```python
from build123d import *

# Parameters (mm, degrees)
SKETCH1_W      = 60
SKETCH1_H      = 60
EXTRUDE1_DEPTH = 50
SKETCH2_W      = 30
SKETCH2_H      = 15
EXTRUDE2_DEPTH = 40
CHAMFER1_SIZE  = 10


with BuildPart() as part:
    # Sketch1 → Extrude1 (new body)
    with BuildSketch(Plane(origin=(0, 0, 0), x_dir=(1, 0, 0), z_dir=(0, 1, 0))):
        Rectangle(SKETCH1_W, SKETCH1_H)
    extrude(amount=EXTRUDE1_DEPTH)

    # Sketch2 → Extrude2 (cut)
    with BuildSketch(Plane(origin=(0, 50, 0), x_dir=(1, 0, 0), z_dir=(0, 1, 0))):
        with Locations((15, -22.5)):
            Rectangle(SKETCH2_W, SKETCH2_H)
    extrude(amount=-EXTRUDE2_DEPTH, mode=Mode.SUBTRACT)

    # Chamfer1
    chamfer1_edges = [part.edges().sort_by_distance(p)[0] for p in [
        (30, 50, -7.5),
    ]]
    chamfer(chamfer1_edges, length=CHAMFER1_SIZE)


solid = part.part
```
Build history of the part. All positions in model axes, mm. A direction names the side the tool comes from. Give positions to 0.01 mm unless a question says otherwise; leave off trailing zeros. Order: outer loops, then holes, each group sorted by start corner. A loop starts at its lowest first (then second) coordinate and runs counter-clockwise, first axis right, second up. Notation, with made-up numbers: M -33.5,-6.75 L 6.5,-6.75 A16 cw 6.5,-1.75 Z; hole C 86.5,0 d11. An arc over 180 degrees is marked long. Write item = value, one per line. Start each with the question number.
(1) Slice it at B-B on x = 9.5. Write the cut outline in (y, z), plus the area to 3 significant figures.
(2) Probe L1, parallel to Z at x = 1, y = 46; L2, parallel to X at y = 21, z = 23; L3, parallel to X at y = 45, z = 7. List the from-to ranges inside material, lowest first. Write a range as [from, to].
(3) Which spindle directions (+Z, -Z, +X, -X, +Y, -Y) get a long thin tool onto all of the face, cutting with end or side? Do faces 1 (the flat face through (30, 20, -6)), 2 (the flat face through (15, 30, 15)). Say none if no direction does.
(4) Slice it at C-C on x = 21. Write the cut outline in (y, z).
(5) Pin check, flat tips, straight feed: pin 1 Ø7.5 at (x, z) = (9, 25.5) entering from +Y; pin 2 Ø7.5 at (y, z) = (25.5, 19) entering from +X; pin 3 Ø12 at (x, y) = (21, 41.5) entering from +Z. Stop position of each tip, or through.
(6) Slice it at A-A on z = -2. Write the cut outline in (x, y).
Responses:
q1.outline = M 0,-30 L 50,-30 L 50,15 L 10,15 L 10,30 L 0,30 Z
q1.area = 2,400 mm2
q2.L1 = [-30, 15]
q2.L2 = [-30, 0]
q2.L3 = [-30, 25]
q3.face_1 = +Z, -Z, +X, +Y, -Y
q3.face_2 = +Z, +X, +Y
q4.outline = M 0,-30 L 49,-30 L 49,15 L 10,15 L 10,30 L 0,30 Z
q5.pin_1 = 10
q5.pin_2 = 0
q5.pin_3 = 15
q6.outline = M -30,0 L 30,0 L 30,40 L 20,50 L -30,50 Z
